Drawing for the job (mm, zero at the part's lowest x, y, z). A direction names the side the tool comes from. Coordinates: 2 decimals unless noted, no trailing zeros. Write each loop counter-clockwise with the first axis right and the second up, starting at its lowest first coordinate (ties: lowest second). Pieces come first, ordered by that corner, then holes. Notation, with made-up numbers: M 71.25,-10.5 L 90.25,-10.5 A19 cw 90.25,-1.5 Z; hole C 72,-31.75 d1. An arc over 180 degrees is marked long. Use a Markdown table: item, result. Add a question column.
Q1. Slice it at C-C on z = 112.5. Write the cut outline in (x, y), then the cut area to 3 significant figures.
Q2. Slice it at B-B on x = 11.5. Write the cut outline in (y, z) (1 decimal).
Q3. Slice it at D-D on y = 141. Write the cut outline in (x, z).
Q4. Wall check: L1, parallel to Y at x = 2.5, z = 93; L2, parallel to Z at x = 16.25, y = 240.5 (1 decimal); L3, parallel to Z at x = 1.5, y = 43. Give the ranges that are in metal, low to high. Write a range as from..to.
Q5. Tool access for the marked faces 1, 2 and 3: list every direction of +Z, -Z, +X, -X, +Y, -Y with a clear straight run to the whole face (end or side of a thin tool).
Q6. Pin check, flat tips, straight feed: pin 1 Ø1 at (x, y) = (15, 159.5) entering from +Z; pin 2 Ø5 at (x, z) = (5, 187) entering from -Y; pin 3 Ø10 at (x, y) = (5.5, 244.5) entering from -Z. Stop position of each tip, or through.
Q7. Slice it at A-A on y = 17. Write the cut outline in (x, z) (1 decimal), then the cut area to 3 significant figures.
Q8. Mould opens along Z. For the marked faces 4, 5 and 6 say: released by +Z, released by -Z, zero draft, split by the parting line, or undercut.
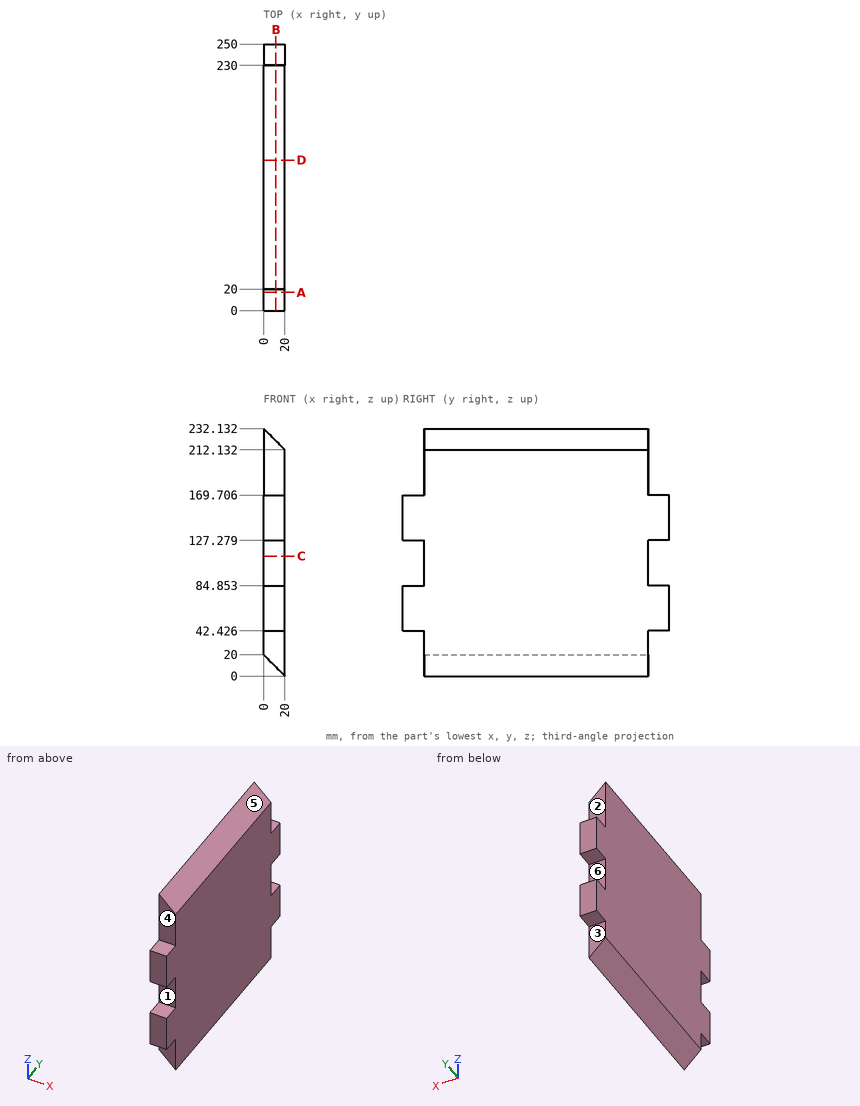
Recorded:
| question | item | result |
|---|---|---|
| 1 | outline | M 0,20 L 20,20 L 20,230 L 0,230 Z |
| 1 | area | 4,200 mm² |
| 2 | outline | M 0,42.4 L 20,42.4 L 20,8.5 L 230,8.5 L 230,42.4 L 250,42.4 L 250,84.9 L 230,84.9 L 230,127.3 L 250,127.3 L 250,169.7 L 230,169.7 L 230,220.6 L 20,220.6 L 20,169.7 L 0,169.7 L 0,127.3 L 20,127.3 L 20,84.9 L 0,84.9 Z |
| 3 | outline | M 0,20 L 20,0 L 20,212.13 L 0,232.13 Z |
| 4 | L1 | 20..230 |
| 4 | L2 | 42.4..84.9, 127.3..169.7 |
| 4 | L3 | 18.5..230.63 |
| 5 | face 1 | +X, -X, -Y |
| 5 | face 2 | +Z, +X, -X, +Y |
| 5 | face 3 | -Z, +X, -X, +Y |
| 6 | pin 1 | z = 217.63 |
| 6 | pin 2 | y = 20 |
| 6 | pin 3 | z = 42.43 |
| 7 | outline | M 0,42.4 L 20,42.4 L 20,84.9 L 0,84.9 Z; M 0,127.3 L 20,127.3 L 20,169.7 L 0,169.7 Z |
| 7 | area | 1,700 mm² |
| 8 | face 4 | zero draft |
| 8 | face 5 | released by +Z |
| 8 | face 6 | undercut |
